Can you work these out from the drawing? Everything is in mm from the part's minimum corner. A direction names the side the tool comes from. Coordinates: 2 decimals unless noted, no trailing zeros. Order: outer loops, then holes, each group sorted by start corner. A loop starts at its lowest first (then second) coordinate and runs counter-clockwise, first axis right, second up. Notation, with made-up numbers: (-6.75, 31.25) -> (42.25, 31.25) arc R32 cw to (42.25, 57.25) -> close; hole circle Ø8 at (18.5, 33). An arc over 180 degrees is marked (long way). Answer in a Markdown table with one row per item.
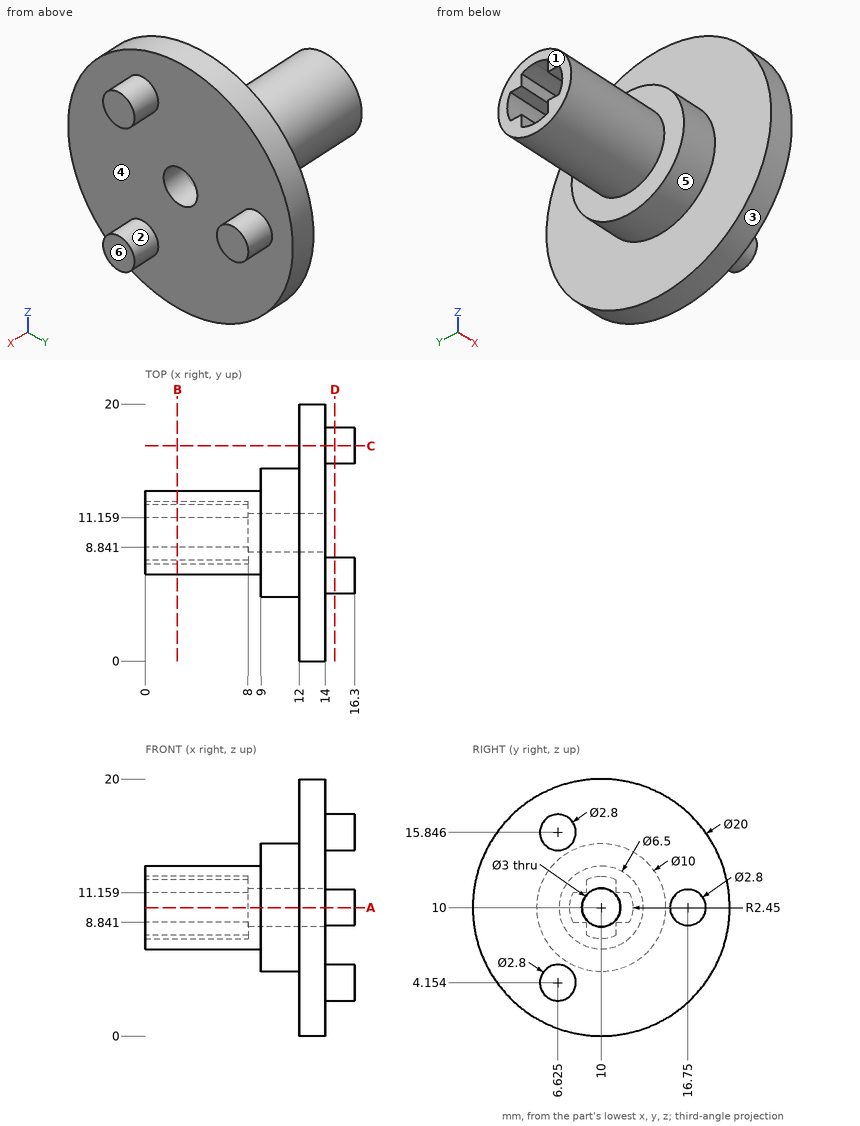
(1) Will these pins go through, and if not, where does the flat tip stop? pin 1 Ø2 at (y, z) = (9.5, 14.5) entering from +X; pin 2 Ø6 at (x, z) = (11.5, 4.5) entering from +Y; pin 3 Ø1.1 at (x, z) = (4.5, 12) entering from -Y.
Response values:
| item | result |
|---|---|
| pin 1 | x = 14 |
| pin 2 | y = 19.67 |
| pin 3 | y = 7.09 |
(2) Suppose I cut it at A-A (z = 10). Please give me the cut outline in (x, y).
Response values:
| item | result |
|---|---|
| outline | (0, 6.75) -> (9, 6.75) -> (9, 5) -> (12, 5) -> (12, 0) -> (14, 0) -> (14, 8.5) -> (8, 8.5) -> (8, 7.55) -> (0, 7.55) -> close; (0, 12.45) -> (8, 12.45) -> (8, 11.5) -> (14, 11.5) -> (14, 15.35) -> (16.3, 15.35) -> (16.3, 18.15) -> (14, 18.15) -> (14, 20) -> (12, 20) -> (12, 15) -> (9, 15) -> (9, 13.25) -> (0, 13.25) -> close |
(3) I need wall thicknesses on line 1 (Y direction, x = 9.15, z = 10); line 2 (Y direction, x = 1.75, z = 10). Which ranges of each line are inside material? Lowest first, please. Write a range as [from, to].
Response values:
| item | result |
|---|---|
| line 1 | [5, 8.5], [11.5, 15] |
| line 2 | [6.75, 7.55], [12.45, 13.25] |
(4) We'd pull the mould along Z, two halves only. Please class the marked faces 1, 2 and 3: +Z half, -Z half, draft (parallel to the pull), parting line (faces both ways), or undercut.
Response values:
| item | result |
|---|---|
| face 1 | draft |
| face 2 | undercut |
| face 3 | parting line |
(5) Suppose I cut it at D-D (x = 14.75). Count the separate pieces of the cut face and the enclosed holes in it, and give its area (3 significant figures).
Response values:
| item | result |
|---|---|
| separate pieces | 3 |
| enclosed holes | 0 |
| area | 18.5 mm2 |
(6) On a 3-axis mill with a long thin cutter (end or side, diameter ignored), from which of +Z, -Z, +X, -X, +Y, -Y can I reach the whole of each face in a straight line? I mean the marked faces 4, 5 and 6. Say none if no direction works.
Response values:
| item | result |
|---|---|
| face 4 | +X |
| face 5 | -X |
| face 6 | +Z, -Z, +X, +Y, -Y |
(7) Suppose I cut it at C-C (y = 16.75). Please give me the cut outline in (x, z).
Response values:
| item | result |
|---|---|
| outline | (12, 2.62) -> (14, 2.62) -> (14, 8.6) -> (16.3, 8.6) -> (16.3, 11.4) -> (14, 11.4) -> (14, 17.38) -> (12, 17.38) -> close |
(8) Suppose I cut it at B-B (x = 2.5). Please give me the cut outline in (y, z), and give its area (3 significant figures).
Response values:
| item | result |
|---|---|
| outline | circle Ø6.5 at (10, 10); hole (7.84, 8.84) -> (8.84, 8.84) -> (8.84, 7.84) arc R2.45 ccw to (11.16, 7.84) -> (11.16, 8.84) -> (12.16, 8.84) arc R2.45 ccw to (12.16, 11.16) -> (11.16, 11.16) -> (11.16, 12.16) arc R2.45 ccw to (8.84, 12.16) -> (8.84, 11.16) -> (7.84, 11.16) arc R2.45 ccw to start |
| area | 16.7 mm2 |
